Could you check a few things on this drawing? It's one solid part, dimensions in mm from its lowest x, y, z. A direction names the side the tool comes from. Round coordinates to 2 decimals unless told otherwise and drop trailing zeros. Loops run counter-clockwise (first coordinate to the right, second up) from the corner with the lowest first, then second, coordinate; pieces in that order, holes last. Notation, with made-up numbers: (11, 60) -> (24, 60) arc R12 ccw to (24, 83) -> close; hole circle Ø3 at (-12.5, -3). An arc over 180 degrees is marked (long way). Put each result on its own line as item: value. Start each with the question number.
1. I need wall thicknesses on line 1 (X direction, y = 16, z = 11); line 2 (Y direction, x = 43.8, z = 15); line 3 (X direction, y = 5, z = 15). Which ranges of each line are inside material? Lowest first, please. Write a range as [from, to].
2. Which directions (+Z, -Z, +X, -X, +Y, -Y) give clear straight access to the entire face, cutting with the end or side of a thin tool? Please do the marked faces 1 and 2.
3. Imagine slicing it at C-C, the plane z = 15. Count the separate pieces of the cut face and the enclosed holes in it, and give its area (3 significant figures).
4. If we mould it in two halves opening along X, with no side actions, what happens to the marked faces 3, 4 and 5? For each: pulls with the +X half, pulls with the -X half, needs draft (parallel to the pull), parting line crosses it, or undercut.
5. Imagine slicing it at A-A, the plane y = 21.5. Please give me the cut outline in (x, z).
6. Imagine slicing it at B-B, the plane x = 22.5. Please give me the cut outline in (y, z), and give its area (3 significant figures).
7. Imagine slicing it at D-D, the plane z = 9.25. Please give me the cut outline in (x, y), and give its area (3 significant figures).
8. I'm going to push flat-ended pins straight in: P1, Ø5, axis at x = 14.5, z = 9.5, coming from the +Y side; P2, Ø8, axis at x = 7, z = 20, coming from the +Y side; P3, Ø3, axis at y = 25, z = 15, coming from the +X side; P4, Ø3, axis at x = 3.5, z = 18, coming from the +Y side. Where does each tip first touch, or does it pass through?
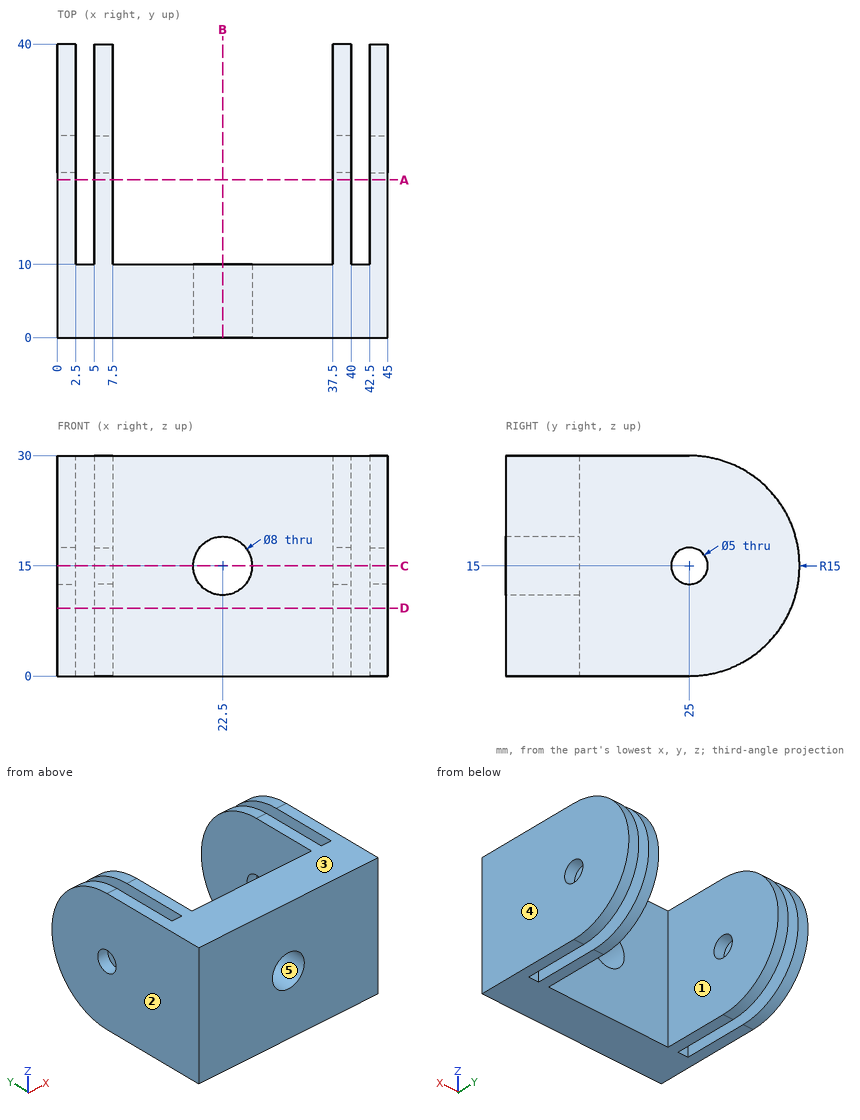
Entries:
1. line 1: [0, 2.5], [5, 7.5], [37.5, 40], [42.5, 45]
1. line 2: [0, 22.5], [27.5, 40]
1. line 3: [0, 18.5], [26.5, 45]
2. face 1: +Z, -Z, +Y
2. face 2: +Z, -Z, -X, +Y, -Y
3. separate pieces: 6
3. enclosed holes: 0
3. area: 620 mm^2
4. face 3: needs draft
4. face 4: pulls with the +X half
4. face 5: undercut
5. outline: (0, 0) -> (2.5, 0) -> (2.5, 30) -> (0, 30) -> close; (5, 0) -> (7.5, 0) -> (7.5, 30) -> (5, 30) -> close; (37.5, 0) -> (40, 0) -> (40, 30) -> (37.5, 30) -> close; (42.5, 0) -> (45, 0) -> (45, 30) -> (42.5, 30) -> close
6. outline: (0, 0) -> (10, 0) -> (10, 11) -> (0, 11) -> close; (0, 19) -> (10, 19) -> (10, 30) -> (0, 30) -> close
6. area: 220 mm^2
7. outline: (0, 0) -> (45, 0) -> (45, 38.85) -> (42.5, 38.85) -> (42.5, 10) -> (40, 10) -> (40, 38.85) -> (37.5, 38.85) -> (37.5, 10) -> (7.5, 10) -> (7.5, 38.85) -> (5, 38.85) -> (5, 10) -> (2.5, 10) -> (2.5, 38.85) -> (0, 38.85) -> close
7. area: 739 mm^2
8. P1: y = 10
8. P2: y = 39.97
8. P3: through
8. P4: y = 39.88
